```python
from build123d import *

# Parameters (mm, degrees)
SKETCH1_W           = 33.5
SKETCH1_H           = 16.85
SKETCH1_R           = 0.95
BOSS_EXTRUDE1_DEPTH = 1.33
SKETCH2_W           = 9.8
SKETCH2_H           = 6.925
BOSS_EXTRUDE2_DEPTH = 10.2


with BuildPart() as part:
    # Sketch1 → Boss-Extrude1 (new body)
    with BuildSketch(Plane.XY):
        Rectangle(SKETCH1_W, SKETCH1_H)
        with Locations((-15, -6.725)):
            Circle(SKETCH1_R, mode=Mode.SUBTRACT)
        with Locations((-15, 6.725)):
            Circle(SKETCH1_R, mode=Mode.SUBTRACT)
    extrude(amount=BOSS_EXTRUDE1_DEPTH)

    # Sketch2 → Boss-Extrude2 (add)
    with BuildSketch(Plane.XY.offset(1.33)):
        with Locations((11.85, 4.9625)):
            Rectangle(SKETCH2_W, SKETCH2_H)
        with Locations((11.85, -4.9625)):
            Rectangle(SKETCH2_W, SKETCH2_H)
    extrude(amount=BOSS_EXTRUDE2_DEPTH)


solid = part.part
```
The model under review builds one solid part; all positions refer to its coordinate system, in mm. A direction names the side the tool comes from. Give positions to 0.01 mm unless a question says otherwise; leave off trailing zeros. Write each loop counter-clockwise with the first axis right and the second up, starting at its lowest first coordinate (ties: lowest second). Pieces come first, ordered by that corner, then holes. Notation, with made-up numbers: (74, 73) -> (104, 73) arc R22 ccw to (104, 89) -> close; hole circle Ø3 at (10, 1). An arc over 180 degrees is marked (long way). Answer in a Markdown table with one row per item.
1) For L1, parallel to Y at x = -15, z = 0.8 (3 decimals); L2, parallel to Y at x = 8.5, z = 8 (3 decimals); L3, parallel to X at y = -7.5, z = 10.75, list the stretches that pass through material, from the lowest coordinate up. Write a range as [from, to].
Worked answers:
| item | result |
|---|---|
| L1 | [-8.425, -7.675], [-5.775, 5.775], [7.675, 8.425] |
| L2 | [-8.425, -1.5], [1.5, 8.425] |
| L3 | [6.95, 16.75] |
2) Tool access review of faces 1 (the flat face through (6.95, 5, 6)), 2 (the flat face through (16.75, -2, 6)), 3 (the flat face through (12, 1.5, 6)): name each direction out of +Z, -Z, +X, -X, +Y, -Y from which nothing blocks a thin tool from reaching the whole face with its end or side.
Worked answers:
| item | result |
|---|---|
| face 1 | +Z, -X, +Y, -Y |
| face 2 | +Z, -Z, +X, +Y, -Y |
| face 3 | +Z, +X, -X |
3) Clearance check with flat-ended pins moving along their axes: P1, Ø3.5, axis at y = -4, z = 7.5, coming from the -X side; P2, Ø3, axis at x = -15, y = 6.725, coming from the -Z side; P3, Ø2, axis at x = -15, y = -6.725, coming from the +Z side. State where each tip first meets the part, or that it passes through.
Worked answers:
| item | result |
|---|---|
| P1 | x = 6.95 |
| P2 | z = 0 |
| P3 | z = 1.33 |
4) Add section D-D on x = 7.5. State the section outline as (y, z) points (3 decimals), plus the area to 3 significant figures.
Worked answers:
| item | result |
|---|---|
| outline | (-8.425, 0) -> (8.425, 0) -> (8.425, 11.53) -> (1.5, 11.53) -> (1.5, 1.33) -> (-1.5, 1.33) -> (-1.5, 11.53) -> (-8.425, 11.53) -> close |
| area | 164 mm² |
5) Add section C-C on y = 4.5. State the section outline as (x, z) points, plus the area to 3 significant figures.
Worked answers:
| item | result |
|---|---|
| outline | (-16.75, 0) -> (16.75, 0) -> (16.75, 11.53) -> (6.95, 11.53) -> (6.95, 1.33) -> (-16.75, 1.33) -> close |
| area | 145 mm² |
6) Mouldability with a two-part tool opening along X and no side actions: class faces 4 (the flat face through (12, -1.5, 6)), 5 (the cylindrical face through (-14.122, -7.089, 0.656)), 6 (the flat face through (-16.75, 0, 1)) as +X half, -X half, draft (parallel to the pull), parting line (faces both ways), or undercut.
Worked answers:
| item | result |
|---|---|
| face 4 | draft |
| face 5 | undercut |
| face 6 | -X half |
7) Add section B-B on z = 9.25. State the section outline as (x, y) points (3 decimals).
Worked answers:
| item | result |
|---|---|
| outline | (6.95, -8.425) -> (16.75, -8.425) -> (16.75, -1.5) -> (6.95, -1.5) -> close; (6.95, 1.5) -> (16.75, 1.5) -> (16.75, 8.425) -> (6.95, 8.425) -> close |
8) Add section A-A on x = -15. State the section outline as (y, z) points (3 decimals), plus the area to 3 significant figures.
Worked answers:
| item | result |
|---|---|
| outline | (-8.425, 0) -> (-7.675, 0) -> (-7.675, 1.33) -> (-8.425, 1.33) -> close; (-5.775, 0) -> (5.775, 0) -> (5.775, 1.33) -> (-5.775, 1.33) -> close; (7.675, 0) -> (8.425, 0) -> (8.425, 1.33) -> (7.675, 1.33) -> close |
| area | 17.4 mm² |
